from build123d import *

# Parameters (mm, degrees)
BOSS_EXTRUDE1_DEPTH     = 37.5
CUT_EXTRUDE1_DEPTH      = 107.548111199
CUT_EXTRUDE1_DEPTH_BACK = 107.548111199
SKETCH2_R               = 11.5
SKETCH2_R_2             = 6.5


with BuildPart() as part:
    # Sketch1 → Boss-Extrude1 (new, symmetric)
    with BuildSketch(Plane(origin=(0, 0, 0), x_dir=(0, 0, -1), z_dir=(1, 0, 0))):
        Polygon((8.5, 21), (8.5, 54), (18.5, 54), (18.5, 21), (18.5, 6.5), (8.5, 6.5), (8.5, 9.648648649), (-8.5, 9.648648649), (-8.5, -9.648648649), (8.5, -9.648648649), (8.5, -6.5), (18.5, -6.5), (18.5, -21), (18.5, -98), (8.5, -98), (8.5, -21), (-18.5, -21), (-18.5, 21), align=None)
    extrude(amount=BOSS_EXTRUDE1_DEPTH, both=True)

    # Sketch2 → Cut-Extrude1 (cut, two sides: drawn at the far end of the back side and taken through both)
    with BuildSketch(Plane.XY.offset(-CUT_EXTRUDE1_DEPTH_BACK)):
        with BuildLine():
            Line((37.5, -98), (37.5, -21))
            Line((37.5, -21), (24.374261359, -78.558361557))
            ThreePointArc((24.374261359, -78.558361557), (15.589114141, -92.544296362), (-6.8e-08, -98))
            Line((-6.8e-08, -98), (37.5, -98))
        make_face()
        with Locations((0, -73)):
            Circle(SKETCH2_R)
        with BuildLine():
            Line((-37.5, -98), (-6.8e-08, -98))
            ThreePointArc((-6.8e-08, -98), (-15.589114194, -92.54429632), (-24.374261359, -78.558361557))
            Line((-24.374261359, -78.558361557), (-37.5, -21))
            Line((-37.5, -21), (-37.5, -98))
        make_face()
        with BuildLine():
            Line((-17.5, -6), (17.5, -6))
            ThreePointArc((17.5, -6), (23.5, 0), (17.5, 6))
            Line((17.5, 6), (-17.5, 6))
            ThreePointArc((-17.5, 6), (-23.5, 0), (-17.5, -6))
        make_face()
        with Locations((24.5, 41)):
            Circle(SKETCH2_R_2)
        with Locations((-24.5, 41)):
            Circle(SKETCH2_R_2)
        with BuildLine():
            Line((37.5, 54), (24.5, 54))
            ThreePointArc((24.5, 54), (33.692388155, 50.192388155), (37.5, 41))
            Line((37.5, 41), (37.5, 54))
        make_face()
        with BuildLine():
            Line((-37.5, 54), (-37.5, 41))
            ThreePointArc((-37.5, 41), (-33.692388155, 50.192388155), (-24.5, 54))
            Line((-24.5, 54), (-37.5, 54))
        make_face()
    extrude(amount=CUT_EXTRUDE1_DEPTH + CUT_EXTRUDE1_DEPTH_BACK, mode=Mode.SUBTRACT)


solid = part.part
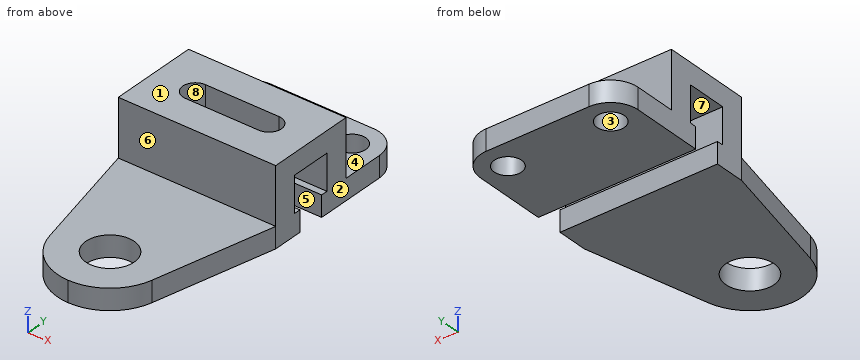
Design review of the part built by this model. Coordinates are the model's own, in mm. Face numbers are marked on the shaded views. A direction names the side the tool comes from. Round coordinates to 2 decimals unless told otherwise and drop trailing zeros. Write each loop counter-clockwise with the first axis right and the second up, starting at its lowest first coordinate (ties: lowest second). Pieces come first, ordered by that corner, then holes.
Item 1: Wall thickness on L1, parallel to Y at x = 0, z = -14.5; L2, parallel to X at y = 41, z = -13.75; L3, parallel to Y at x = 6, z = 15: over which ranges is each line inside the solid? List them lowest first.
Item 2: Consider section A-A on y = 0. Give the boundary of the cut face in (x, z).
Item 3: Consider section B-B on z = 0. Give the boundary of the cut face in (x, y).
Item 4: Consider section D-D on x = 29. Give the boundary of the cut face in (y, z).
Item 5: Consider section C-C on x = 19.5. Give the boundary of the cut face in (y, z).
Item 6: For the marked faces 4, 5, 6, 7 and 8, list the 3-axis set-ups (+Z, -Z, +X, -X, +Y, -Y) from which the entire face can be reached by the end or side of a thin tool; tool diameter is ignored.
Item 7: For pin 1 Ø5 at (x, z) = (-4.5, 15.5) entering from -Y; pin 2 Ø6 at (x, y) = (-21, -79) entering from +Z; pin 3 Ø12 at (y, z) = (-53, -8.5) entering from -X, all flat-tipped, find the tip position at first contact; note any pin that passes through.
Item 8: Draft analysis for pull direction X (two halves, no side actions). For the marked faces 1, 2 and 3, state which applies: released by +X, released by -X, zero draft, split by the parting line, or undercut.
Check values:
1. L1: y = -98 to -84.5, -61.5 to -6.5, 6.5 to 54
1. L2: x = -37.5 to -31, -18 to 18, 31 to 37.5
1. L3: y = -21 to -6, 6 to 21
2. outline: (-37.5, 8.5) - (-23.5, 8.5) - (-23.5, 18.5) - (-37.5, 18.5) - close; (23.5, 8.5) - (37.5, 8.5) - (37.5, 18.5) - (23.5, 18.5) - close
3. outline: (-37.5, -21) - (37.5, -21) - (37.5, -9.65) - (-37.5, -9.65) - close; (-37.5, 9.65) - (37.5, 9.65) - (37.5, 21) - (-37.5, 21) - close
4. outline: (-58.27, -18.5) - (-6.5, -18.5) - (-6.5, -8.5) - (-9.65, -8.5) - (-9.65, 8.5) - (9.65, 8.5) - (9.65, -8.5) - (6.5, -8.5) - (6.5, -18.5) - (36.31, -18.5) - (36.31, -8.5) - (21, -8.5) - (21, 18.5) - (-21, 18.5) - (-21, -8.5) - (-58.27, -8.5) - close; (45.69, -18.5) - (53.2, -18.5) - (53.2, -8.5) - (45.69, -8.5) - close
5. outline: (-88.64, -18.5) - (-6.5, -18.5) - (-6.5, -8.5) - (-9.65, -8.5) - (-9.65, 8.5) - (-5.66, 8.5) - (-5.66, 18.5) - (-21, 18.5) - (-21, -8.5) - (-88.64, -8.5) - close; (5.66, 8.5) - (9.65, 8.5) - (9.65, -8.5) - (6.5, -8.5) - (6.5, -18.5) - (36.85, -18.5) - (36.85, -8.5) - (21, -8.5) - (21, 18.5) - (5.66, 18.5) - close; (45.15, -18.5) - (54, -18.5) - (54, -8.5) - (45.15, -8.5) - close
6. face 4: +Z, +X, -X, +Y
6. face 5: -Z, +X, -X
6. face 6: +Z, +X, -X, -Y
6. face 7: +X, -X
6. face 8: +Z, -Z
7. pin 1: stops at y = -21
7. pin 2: stops at z = -8.5
7. pin 3: stops at x = -31.57
8. face 1: zero draft
8. face 2: released by +X
8. face 3: undercut
